Geometry: see drawing. Coordinates: mm, zero at the bounding-box minimum. A direction names the side the tool comes from. Coordinates: 2 decimals unless noted, no trailing zeros. Loops run counter-clockwise (first coordinate to the right, second up) from the corner with the lowest first, then second, coordinate; pieces in that order, holes last. Notation, with made-up numbers: (-29, 81.25) -> (28, 81.25) arc R30 ccw to (28, 117.25) -> close; hole circle Ø10 at (-36.5, 39.25). An arc over 180 degrees is marked (long way). Answer as a JSON object with one key per item and string values.
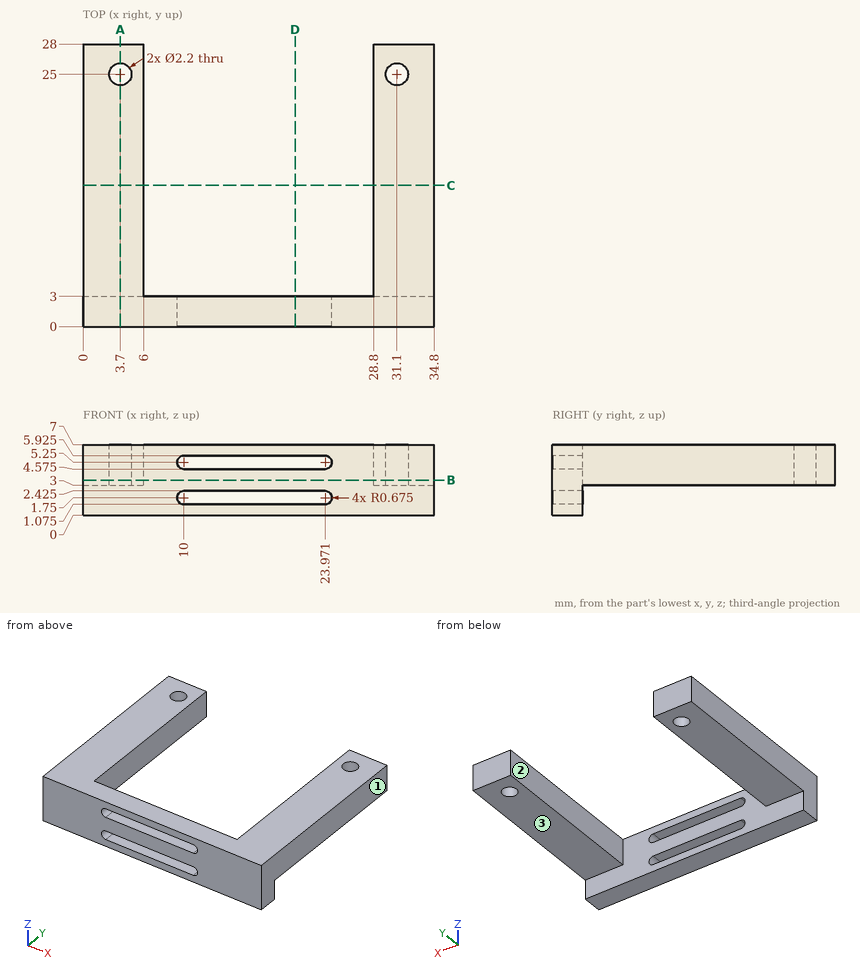
1. Section query C-C (y = 14). Return loops of the section in (x, z), plus the area to 3 significant figures.
Reply:
{"outline": "(0, 3) -> (6, 3) -> (6, 7) -> (0, 7) -> close; (28.8, 3) -> (34.8, 3) -> (34.8, 7) -> (28.8, 7) -> close", "area": "48.0 mm2"}
2. Access query for the marked faces 1, 2 and 3. Directions: +Z, -Z, +X, -X, +Y, -Y. A direction counts if a zero-diameter tool reaches every point of the face in a straight line with its end or side. Return the directions, or none.
Reply:
{"face 1": "+Z, -Z, +X, +Y, -Y", "face 2": "+Z, -Z, +Y", "face 3": "-Z, +X, -X, +Y"}
3. Section query B-B (z = 3.5). Return loops of the section in (x, y), plus the area to 3 significant figures.
Reply:
{"outline": "(0, 0) -> (34.8, 0) -> (34.8, 28) -> (28.8, 28) -> (28.8, 3) -> (6, 3) -> (6, 28) -> (0, 28) -> close; hole circle Ø2.2 at (3.7, 25); hole circle Ø2.2 at (31.1, 25)", "area": "397 mm2"}
4. Line query: line 1 along Y through (x, z) = (3.7, 4.85); line 2 along X through (y, z) = (13.5, 6); line 3 along Y through (x, z) = (8, 4.75). Output: solid intervals per line, ascending.
Reply:
{"line 1": "y = 0 to 23.9, 26.1 to 28", "line 2": "x = 0 to 6, 28.8 to 34.8", "line 3": "y = 0 to 3"}
5. Section query A-A (x = 3.7). Return loops of the section in (y, z), plus the area to 3 significant figures.
Reply:
{"outline": "(0, 0) -> (3, 0) -> (3, 3) -> (23.9, 3) -> (23.9, 7) -> (0, 7) -> close; (26.1, 3) -> (28, 3) -> (28, 7) -> (26.1, 7) -> close", "area": "112 mm2"}
6. Section query D-D (x = 21). Return loops of the section in (y, z) (1 decimal).
Reply:
{"outline": "(0, 0) -> (3, 0) -> (3, 1.1) -> (0, 1.1) -> close; (0, 2.4) -> (3, 2.4) -> (3, 4.6) -> (0, 4.6) -> close; (0, 5.9) -> (3, 5.9) -> (3, 7) -> (0, 7) -> close"}
7. Pin query (flat end, axial travel): P1, Ø3, axis at x = 31.5, y = 19.5, coming from the -Z side; P2, Ø2, axis at x = 15.5, z = 5, coming from the +Y side. Return the tip coordinate at first contact, or that it passes through.
Reply:
{"P1": "stops at z = 3", "P2": "stops at y = 3"}
